from build123d import *

# Parameters (mm, degrees)
F0_R     = 8.5
F1_DEPTH = 4
F2_R     = 5
F3_DEPTH = 100


with BuildPart() as f1:
    # F0 (on Top) → F1 (new body)
    with BuildSketch(Plane.XY):
        Circle(F0_R)
    extrude(amount=F1_DEPTH)

    # F2 (on Top) → F3 (join)
    with BuildSketch(Plane.XY):
        Circle(F2_R)
    extrude(amount=F3_DEPTH)

    # F4 (on Right) → F5 (revolve)
    with BuildSketch(Plane.YZ):
        Polygon((3, 105), (0, 105), (0, 100), (4, 100), align=None)
    revolve(axis=Axis((0, 0, 102.5), (0, 0, -1)))

    # F6 (on Right) → F7 (revolve)
    with BuildSketch(Plane.YZ):
        Polygon((1, 110), (0, 110), (0, 105), (2, 105), align=None)
    revolve(axis=Axis((0, 0, 107.5), (0, 0, -1)))


solid = f1.part
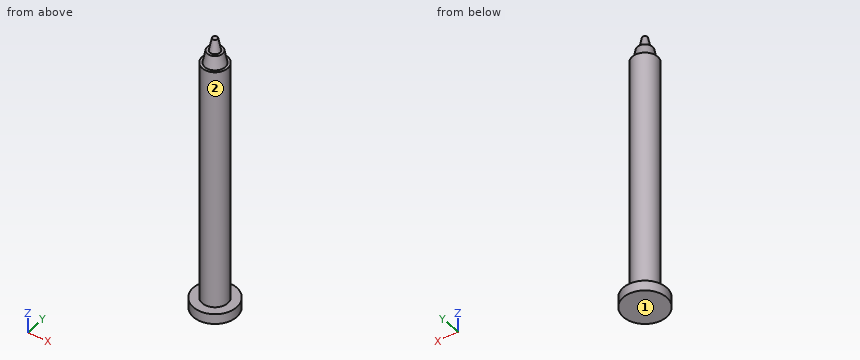
The model under review builds one solid part; all positions refer to its coordinate system, in mm. Face numbers are marked on the shaded views. A direction names the side the tool comes from. Coordinates: 2 decimals unless noted, no trailing zeros. Loops run counter-clockwise (first coordinate to the right, second up) from the corner with the lowest first, then second, coordinate; pieces in that order, holes last. Notation, with made-up numbers: (25, 76.5) -> (38, 76.5) arc R22 cw to (38, 104.5) -> close; hole circle Ø8 at (83.25, -35.75). An arc over 180 degrees is marked (long way). Use a Markdown table: item, result. Add a question column.
1. Add section D-D on x = -6. Write out the cut boundary in (y, z).
2. Machinability: for the marked faces 1 and 2, which of the approach directions +Z, -Z, +X, -X, +Y, -Y give a long, thin tool a straight path to every point of the face, cutting with its end or side? Answer none if there is none.
3. Clearance check with flat-ended pins moving along their axes: pin 1 Ø1 at (y, z) = (-5, 87) entering from -X; pin 2 Ø5 at (y, z) = (6, 74) entering from +X; pin 3 Ø2 at (x, y) = (3.5, 1) entering from +Z. State where each tip first meets the part, or that it passes through.
4. Add section C-C on z = 70.5. Write out the cut boundary in (x, y), plus the area to 3 significant figures.
5. Add section A-A on y = 0. Write out the cut boundary in (x, z), plus the area to 3 significant figures.
6. To check wall thickness, follow line 1 (Z direction, x = 2.5, y = 5.75); line 2 (Z direction, x = 4.25, y = -0.5); line 3 (Y direction, x = -0.25, z = 50). State the ranges of each line that lie inside material, in increasing order.
Returned:
| question | item | result |
|---|---|---|
| 1 | outline | (-6.02, 0) -> (6.02, 0) -> (6.02, 4) -> (-6.02, 4) -> close |
| 2 | face 1 | -Z, +X, -X, +Y, -Y |
| 2 | face 2 | +Z |
| 3 | pin 1 | stops at x = -2.18 |
| 3 | pin 2 | stops at x = 3.57 |
| 3 | pin 3 | stops at z = 105 |
| 4 | outline | circle Ø10 at (0, 0) |
| 4 | area | 78.5 mm² |
| 5 | outline | (-8.5, 0) -> (8.5, 0) -> (8.5, 4) -> (5, 4) -> (5, 100) -> (4, 100) -> (3, 105) -> (2, 105) -> (1, 110) -> (-1, 110) -> (-2, 105) -> (-3, 105) -> (-4, 100) -> (-5, 100) -> (-5, 4) -> (-8.5, 4) -> close |
| 5 | area | 1,080 mm² |
| 6 | line 1 | z = 0 to 4 |
| 6 | line 2 | z = 0 to 100 |
| 6 | line 3 | y = -4.99 to 4.99 |
